Design review of the part built by this model. Coordinates are the model's own, in mm. Face numbers are marked on the shaded views. A direction names the side the tool comes from. Give positions to 0.01 mm unless a question says otherwise; leave off trailing zeros. Loops run counter-clockwise (first coordinate to the right, second up) from the corner with the lowest first, then second, coordinate; pieces in that order, holes last. Notation, with made-up numbers: (10.25, 86.25) - (22.25, 86.25) arc R5 ccw to (22.25, 92.25) - close; hole circle Ø8 at (58, 49). An arc over 180 degrees is marked (long way). One line per item, written item: value. Start each with the question number.
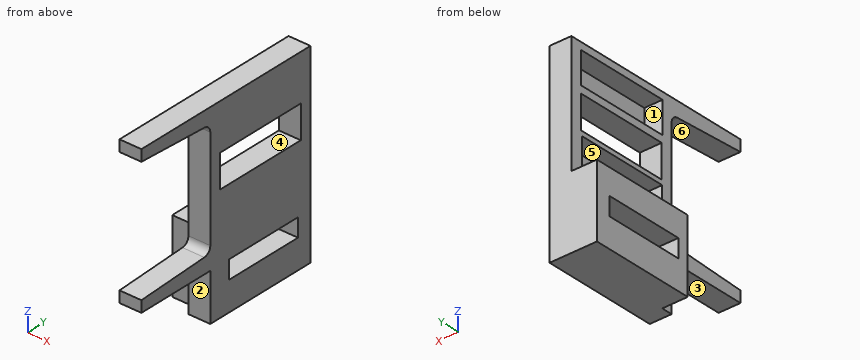
```python
from build123d import *

# Parameters (mm, degrees)
SKETCH1_W           = 53
SKETCH1_H           = 32
BOSS_EXTRUDE1_DEPTH = 13
SKETCH7_W           = 7
SKETCH7_H           = 40
CUT_EXTRUDE3_DEPTH  = 44.534469102
SKETCH8_W           = 6
SKETCH8_H           = 40
BOSS_EXTRUDE2_DEPTH = 22
SKETCH20_W          = 6
SKETCH20_H          = 31.5
CUT_EXTRUDE9_DEPTH  = 44.534469102
CUT_EXTRUDE9_DRAFT  = -3
FILLET1_R           = 2
FILLET2_R           = 2
SKETCH49_W          = 7
SKETCH49_H          = 32
BOSS_EXTRUDE3_DEPTH = 7
SKETCH50_W          = 7
SKETCH50_H          = 20
CUT_EXTRUDE19_DEPTH = 3
SKETCH35_W          = 9
SKETCH35_H          = 25.742086546
CUT_EXTRUDE15_DEPTH = 47.853495067
SKETCH36_W          = 8.51187264
SKETCH36_H          = 25.698199293
CUT_EXTRUDE16_DEPTH = 5
SKETCH55_W          = 8.650111134
SKETCH55_H          = 26.010357873
CUT_EXTRUDE20_DEPTH = 5
SKETCH63_W          = 5
SKETCH63_H          = 22
CUT_EXTRUDE21_DEPTH = 49.117044797


with BuildPart() as part:
    # Sketch1 → Boss-Extrude1 (new body)
    with BuildSketch(Plane(origin=(0, 0, 0), x_dir=(0, 0, -1), z_dir=(1, 0, 0))):
        Rectangle(SKETCH1_W, SKETCH1_H)
    extrude(amount=BOSS_EXTRUDE1_DEPTH)

    # Sketch7 → Cut-Extrude3 (cut, through all)
    with BuildSketch(Plane(origin=(0, 16, 0), x_dir=(1, 0, 0), z_dir=(0, 1, 0))):
        with Locations((3.5, 6.5)):
            Rectangle(SKETCH7_W, SKETCH7_H)
    extrude(amount=-CUT_EXTRUDE3_DEPTH, mode=Mode.SUBTRACT)

    # Sketch8 → Boss-Extrude2 (add)
    with BuildSketch(Plane.XZ.offset(16)):
        with Locations((10, -6.5)):
            Rectangle(SKETCH8_W, SKETCH8_H)
    extrude(amount=BOSS_EXTRUDE2_DEPTH)


with BuildPart() as cut_extrude9_tool:
    # Sketch20 → Cut-Extrude9 (with draft: the straight prism first)
    with BuildSketch(Plane(origin=(0, -16, 0), x_dir=(-1, 0, 0), z_dir=(0, -1, 0))):
        with Locations((-10, 6.5)):
            Rectangle(SKETCH20_W, SKETCH20_H)
    extrude(amount=CUT_EXTRUDE9_DEPTH)
    # Cut-Extrude9: the draft: its side faces are tilted about the plane it starts from
    cut_extrude9_sides = [cut_extrude9_tool.faces().sort_by_distance(p)[0] for p in [
        (10, -38.267234551, 9.25),
        (7, -38.267234551, -6.5),
        (10, -38.267234551, -22.25),
        (13, -38.267234551, -6.5),
    ]]
    draft(cut_extrude9_sides, Plane(origin=(0, -16, 0), x_dir=(-1, 0, 0), z_dir=(0, -1, 0)), CUT_EXTRUDE9_DRAFT)


with BuildPart() as part_1:
    add(part.part)

    # Cut-Extrude9: cut by cut_extrude9_tool
    add(cut_extrude9_tool.part, mode=Mode.SUBTRACT)

    # Fillet1
    fillet1_edges = [part_1.edges().sort_by_distance(p)[0] for p in [
        (10, -16, -22.25),
    ]]
    fillet(fillet1_edges, radius=FILLET1_R)

    # Fillet2
    fillet2_edges = [part_1.edges().sort_by_distance(p)[0] for p in [
        (10, -16, 9.25),
    ]]
    fillet(fillet2_edges, radius=FILLET2_R)

    # Sketch49 → Boss-Extrude3 (add)
    with BuildSketch(Plane(origin=(0, 0, 13.5), x_dir=(-1, 0, 0), z_dir=(0, 0, -1))):
        with Locations((-3.5, 0)):
            Rectangle(SKETCH49_W, SKETCH49_H)
    extrude(amount=BOSS_EXTRUDE3_DEPTH)

    # Sketch50 → Cut-Extrude19 (cut)
    with BuildSketch(Plane.XZ.offset(16)):
        with Locations((3.5, 16.5)):
            Rectangle(SKETCH50_W, SKETCH50_H)
    extrude(amount=-CUT_EXTRUDE19_DEPTH, mode=Mode.SUBTRACT)

    # Sketch35 → Cut-Extrude15 (cut, through all)
    with BuildSketch(Plane.ZY.offset(-7)):
        with Locations((-9.381446742, 0.030527838)):
            Rectangle(SKETCH35_W, SKETCH35_H)
    extrude(amount=-CUT_EXTRUDE15_DEPTH, mode=Mode.SUBTRACT)

    # Sketch36 → Cut-Extrude16 (cut)
    with BuildSketch(Plane.ZY.offset(-7)):
        with Locations((0.636992311, -0.150900353)):
            Rectangle(SKETCH36_W, SKETCH36_H)
    extrude(amount=-CUT_EXTRUDE16_DEPTH, mode=Mode.SUBTRACT)

    # Sketch55 → Cut-Extrude20 (cut)
    with BuildSketch(Plane.ZY.offset(-7)):
        with Locations((-20.206502309, -0.103607826)):
            Rectangle(SKETCH55_W, SKETCH55_H)
    extrude(amount=-CUT_EXTRUDE20_DEPTH, mode=Mode.SUBTRACT)

    # Sketch63 → Cut-Extrude21 (cut, through all)
    with BuildSketch(Plane.ZY):
        with Locations((16, 1)):
            Rectangle(SKETCH63_W, SKETCH63_H)
    extrude(amount=-CUT_EXTRUDE21_DEPTH, mode=Mode.SUBTRACT)


with BuildPart() as body_2:
    # Mirror1: mirrored copy
    add(part_1.part.mirror(Plane(origin=(13, 16, 26.5), x_dir=(1, 0, 0), z_dir=(0, 0, -1))))


solid = body_2.part
```
(1) Take a section at A-A on z = 60. State the section outline as (x, y) points, and give its area (3 significant figures).
(2) Machinability: for the marked faces 4, 5 and 6, which of the approach directions +Z, -Z, +X, -X, +Y, -Y give a long, thin tool a straight path to every point of the face, cutting with its end or side? Answer none if there is none.
(3) Draft analysis for pull direction Z (two halves, no side actions). For the marked faces 1, 2 and 3, state which applies: pulls with the +Z half, pulls with the -Z half, needs draft (parallel to the pull), parting line crosses it, or undercut.
(4) To check wall thickness, follow L1, parallel to Z at x = 11, y = -8; L2, parallel to Z at x = 3.5, y = -9; L3, parallel to Y at x = 8.25, z = 53. State the ranges of each line that lie inside material, in increasing order. Write a range as from..to.
(5) Take a section at D-D on x = 10. State the section outline as (y, z) points, and give its area (3 significant figures).
(6) Take a section at B-B on x = 3. State the section outline as (y, z) points.
(7) For pin 1 Ø2.5 at (x, z) = (4, 36.5) entering from -Y; pin 2 Ø3 at (x, z) = (10.5, 33.5) entering from -Y; pin 3 Ø12 at (y, z) = (-1, 62.5) entering from -X, all flat-tipped, find the tip position at first contact; note any pin that passes through.
(8) Take a section at C-C on y = -7. State the section outline as (x, z) points, and give its area (3 significant figures).
Here are the results:
1. outline: (7, -16) - (13, -16) - (13, -12.84) - (7, -12.84) - close; (7, 12.9) - (13, 12.9) - (13, 16) - (7, 16) - close
1. area: 37.5 mm²
2. face 4: +X, -X
2. face 5: -X
2. face 6: +X, -X, -Y
3. face 1: undercut
3. face 2: needs draft
3. face 3: pulls with the -Z half
4. L1: 26.5..34.5, 39.5..48.11, 56.62..57.88, 66.88..68.88, 77.53..79.5
4. L2: 26.5..34.5, 39.5..46.5
4. L3: -16..-13, 12.7..16
5. outline: (-38, 39.5) - (-16, 39.5) - (-16, 26.5) - (16, 26.5) - (16, 79.5) - (-38, 79.5) - (-38, 76.4) - (-17.9, 75.35) arc R2 cw to (-16, 73.35) - (-16, 45.65) arc R2 cw to (-17.9, 43.65) - (-38, 42.6) - close; hole (-13.11, 68.88) - (12.9, 68.88) - (12.9, 77.53) - (-13.11, 77.53) - close; hole (-13, 48.11) - (12.7, 48.11) - (12.7, 56.62) - (-13, 56.62) - close; hole (-12.84, 57.88) - (12.9, 57.88) - (12.9, 66.88) - (-12.84, 66.88) - close; hole (-10, 34.5) - (12, 34.5) - (12, 39.5) - (-10, 39.5) - close
5. area: 1,070 mm²
6. outline: (-13, 26.5) - (16, 26.5) - (16, 46.5) - (-13, 46.5) - close; hole (-10, 34.5) - (12, 34.5) - (12, 39.5) - (-10, 39.5) - close
7. pin 1: y = -13
7. pin 2: y = -16
7. pin 3: x = 7
8. outline: (0, 26.5) - (13, 26.5) - (13, 34.5) - (0, 34.5) - close; (0, 39.5) - (13, 39.5) - (13, 57.88) - (7, 57.88) - (7, 56.62) - (12, 56.62) - (12, 48.11) - (7, 48.11) - (7, 46.5) - (0, 46.5) - close; (7, 66.88) - (13, 66.88) - (13, 79.5) - (7, 79.5) - (7, 77.53) - (12, 77.53) - (12, 68.88) - (7, 68.88) - close
8. area: 253 mm²
